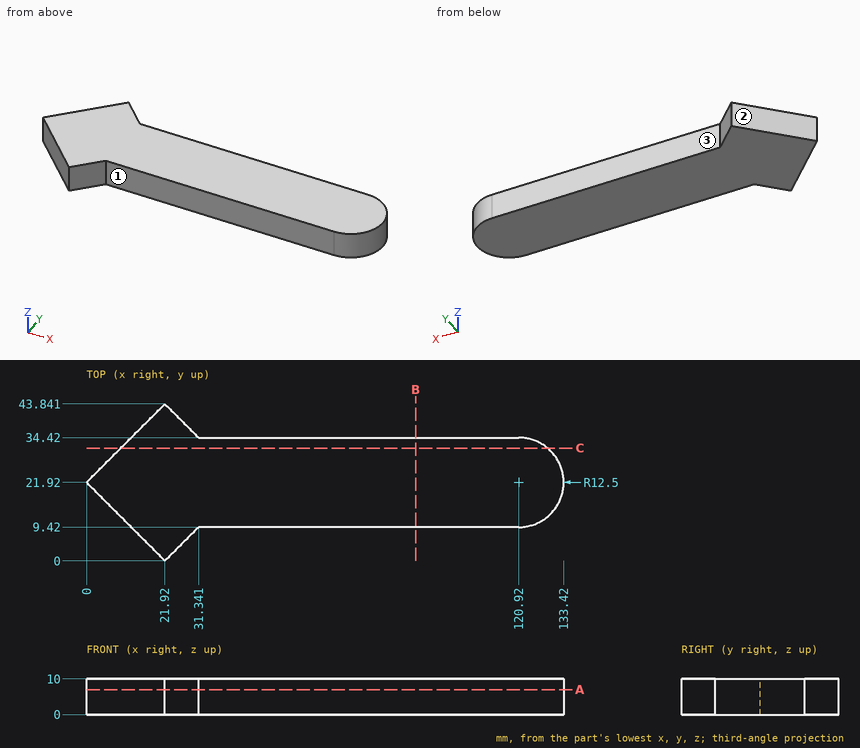
Here's the drawing with two shaded views (mm, measured from the low corner). I have some questions. A direction names the side the tool comes from. Give positions to 0.01 mm unless a question says otherwise; leave off trailing zeros. Order: outer loops, then holes, each group sorted by start corner. A loop starts at its lowest first (then second) coordinate and runs counter-clockwise, first axis right, second up. Notation, with made-up numbers: (26.25, 79) - (44.25, 79) arc R28 cw to (44.25, 113) - close; hole circle Ø2 at (20, 82). An arc over 180 degrees is marked (long way). Use a Markdown table: item, result. Add a question column.
Q1. On a 3-axis mill with a long thin cutter (end or side, diameter ignored), from which of +Z, -Z, +X, -X, +Y, -Y can I reach the whole of each face in a straight line? I mean the marked faces 1, 2 and 3. Say none if no direction works.
Q2. If we section it at C-C on y = 31.5: Write out the boundary of the cut face in (x, z).
Q3. If we section it at A-A on z = 7: Write out the boundary of the cut face in (x, y), plus the area to 3 significant figures.
Q4. If we section it at B-B on x = 92: Write out the boundary of the cut face in (y, z), plus the area to 3 significant figures.
Q5. I'm going to push flat-ended pins straight in: pin 1 (1 mm diameter, centred on x = 41.5, z = 1.5, fed in from -Y); pin 2 (2 mm diameter, centred on x = 13.5, z = 2, fed in from -Y); pin 3 (2 mm diameter, centred on x = 32, z = 6, fed in from -Y). Where does each tip first touch, or does it pass through?
Q6. Please list where these lines run through material, in increasing order: line 1 along Y through (x, z) = (96, 2); line 2 along X through (y, z) = (38.5, 8.5); line 3 along X through (y, z) = (42.5, 5.25).
Answers follow:
| question | item | result |
|---|---|---|
| 1 | face 1 | +Z, -Z, +X, -Y |
| 1 | face 2 | +Z, -Z, -X, +Y |
| 1 | face 3 | +Z, -Z, +X, +Y |
| 2 | outline | (9.58, 0) - (128.95, 0) - (128.95, 10) - (9.58, 10) - close |
| 3 | outline | (0, 21.92) - (21.92, 0) - (31.34, 9.42) - (120.92, 9.42) arc R12.5 ccw to (120.92, 34.42) - (31.34, 34.42) - (21.92, 43.84) - close |
| 3 | area | 3,290 mm^2 |
| 4 | outline | (9.42, 0) - (34.42, 0) - (34.42, 10) - (9.42, 10) - close |
| 4 | area | 250 mm^2 |
| 5 | pin 1 | stops at y = 9.42 |
| 5 | pin 2 | stops at y = 7.42 |
| 5 | pin 3 | stops at y = 9.08 |
| 6 | line 1 | y = 9.42 to 34.42 |
| 6 | line 2 | x = 16.58 to 27.26 |
| 6 | line 3 | x = 20.58 to 23.26 |
